from build123d import *
from build123d.topology import SkipClean

# Parameters (mm, degrees)
SKETCH_1_R          = 24.5
EXTRUDE_1_DEPTH     = 4.75
EXTRUDE_START       = 5.5
EXTRUDE_2_DEPTH     = 5.5
EXTRUDE_START_2     = 4.75
EXTRUDE_3_DEPTH     = 4.75
SKETCH_6_R          = 8.95
CUT_EXTRUDE_1_DEPTH = 38.755794257
SKETCH_8_W          = 30
SKETCH_8_H          = 10
EXTRUDE_4_DEPTH     = 5
FILLET_1_R          = 10
FILLET_2_R          = 5
MM_1_D              = 5
SKETCH_11_W         = 11.168523271
SKETCH_11_H         = 1.926491066
CUT_EXTRUDE_2_DEPTH = 45.650628903
CUT_EXTRUDE_3_DEPTH = 45.584890939
FILLET_3_R          = 2.5


# Some blends are built 0.0001 mm under size
with BuildPart() as part:
    # 草图1 → 凸台-拉伸1 (new body)
    with BuildSketch(Plane(origin=(0, 0, 0), x_dir=(1, 0, 0), z_dir=(0, 1, 0))):
        with Locations(Location((0, 0, 0), (0, 0, 270))):
            Circle(SKETCH_1_R)
    extrude(amount=EXTRUDE_1_DEPTH)

    # 草图4 → 凸台-拉伸2 (add)
    with BuildSketch(Plane.XZ.offset(EXTRUDE_START)):
        with BuildLine():
            Line((-23, 0), (-24.5, 0))
            ThreePointArc((-24.5, 0), (-22.635048547, 9.375744093), (-17.324116139, 17.324116139))
            Line((-17.324116139, 17.324116139), (-16.263455967, 16.263455967))
            ThreePointArc((-16.263455967, 16.263455967), (-21.249229248, 8.801718944), (-23, 0))
        make_face()
        with BuildLine():
            Line((23, 0), (24.5, 0))
            ThreePointArc((24.5, 0), (22.635048547, -9.375744093), (17.324116139, -17.324116139))
            Line((17.324116139, -17.324116139), (16.263455967, -16.263455967))
            ThreePointArc((16.263455967, -16.263455967), (21.249229248, -8.801718944), (23, 0))
        make_face()
    extrude(amount=-EXTRUDE_2_DEPTH)

    # 草图5 → 凸台-拉伸3 (add)
    with SkipClean():  # the faces are left unmerged after this step: merging them gives an invalid solid
        with BuildSketch(Plane.XZ.offset(5.5).offset(EXTRUDE_START_2)):
            with BuildLine():
                Line((-23, 0), (-24.5, 0))
                ThreePointArc((-24.5, 0), (-18.768088856, 15.748296437), (-4.254380353, 24.127789949))
                Line((-4.254380353, 24.127789949), (-3.993908086, 22.650578319))
                ThreePointArc((-3.993908086, 22.650578319), (-17.619022192, 14.784115023), (-23, 0))
            make_face()
            with BuildLine():
                Line((3.993908086, -22.650578319), (4.254380353, -24.127789949))
                ThreePointArc((4.254380353, -24.127789949), (18.768088856, -15.748296437), (24.5, 0))
                Line((24.5, 0), (23, 0))
                ThreePointArc((23, 0), (17.619022192, -14.784115023), (3.993908086, -22.650578319))
            make_face()
        extrude(amount=-EXTRUDE_3_DEPTH)

    # 草图6 → 切除-拉伸1 (cut, through all)
    with SkipClean():  # the faces are left unmerged after this step: merging them gives an invalid solid
        with BuildSketch(Plane(origin=(0, 4.75, 0), x_dir=(1, 0, 0), z_dir=(0, 1, 0))):
            with Locations(Location((0, 0, 0), (0, 0, 270))):
                Circle(SKETCH_6_R)
        extrude(amount=-CUT_EXTRUDE_1_DEPTH, mode=Mode.SUBTRACT)

    # 草图8 → 凸台-拉伸4 (add)
    with SkipClean():  # the faces are left unmerged after this step: merging them gives an invalid solid
        with BuildSketch(Plane(origin=(0, 0, 0), x_dir=(0.7071067811865489, 0, -0.7071067811865462), z_dir=(0.7071067811865462, 0, 0.7071067811865489))):
            with Locations((24.5, 9.75)):
                Rectangle(SKETCH_8_W, SKETCH_8_H)
        extrude(amount=EXTRUDE_4_DEPTH)

    # 圆角1
    fillet_1_edges = [part.edges().sort_by_distance(p)[0] for p in [
        (8.485281374, 14.75, -4.949747468),
    ]]
    fillet(fillet_1_edges, radius=FILLET_1_R - 0.0001)  # a hair under: the kernel refuses the full size

    # 圆角2
    fillet_2_edges = [part.edges().sort_by_distance(p)[0] for p in [
        (29.69848481, 14.75, -26.162950904),
        (29.69848481, 4.75, -26.162950904),
    ]]
    fillet(fillet_2_edges, radius=FILLET_2_R - 0.0001)  # a hair under: the kernel refuses the full size

    # 大小mm 暗销孔1 (through all)
    with Locations(Plane(origin=(3.535533906, 0, 3.535533906), x_dir=(0.7071067811865488, 0, -0.7071067811865462), z_dir=(0.7071067811865462, 0, 0.7071067811865488))):
        with Locations((32.49436991, 9.75)):
            Hole(MM_1_D / 2)

    # 草图11 → 切除-拉伸2 (cut, through all)
    with BuildSketch(Plane(origin=(3.535533906, 0, 3.535533906), x_dir=(0.7071067811865489, 0, -0.7071067811865461), z_dir=(0.7071067811865461, 0, 0.7071067811865489))):
        with Locations((29.568631546, 5.713245533)):
            Rectangle(SKETCH_11_W, SKETCH_11_H)
    extrude(amount=-CUT_EXTRUDE_2_DEPTH, mode=Mode.SUBTRACT)

    # 草图12 → 切除-拉伸3 (cut, through all)
    with BuildSketch(Plane(origin=(0, 0, 0), x_dir=(-0.7071067811865489, 0, 0.7071067811865461), z_dir=(-0.7071067811865461, 0, -0.7071067811865489))):
        with BuildLine():
            Line((-32.081510731, 14.75), (-9.5, 4.75))
            ThreePointArc((-9.5, 4.75), (-12.428932188, 11.821067812), (-19.5, 14.75))
            Line((-19.5, 14.75), (-32.081510731, 14.75))
        make_face()
    extrude(amount=-CUT_EXTRUDE_3_DEPTH, mode=Mode.SUBTRACT)


with BuildPart() as cut_extrude_3_kept_piece:
    # of the separate pieces the step leaves, the one the design keeps (cut_extrude_3_pieces_kept)
    add(part.part.solids().sort_by_distance((24.395254662, 14.75, -24.395254662))[0])

    # 圆角3
    # the kernel refuses this fillet: 2.5 mm, written as the material it takes off along each edge
    with BuildSketch(Plane(origin=(-16.75, -10.25, 0), x_dir=(0, 1, 0), z_dir=(-1, 0, 0)), Plane(origin=(2.908606976, -10.25, -16.495529863), x_dir=(0.9848077530122085, 0, 0.17364817766692725), z_dir=(0.17364817766692725, 0, -0.9848077530122086)), Plane(origin=(30.75, -10.25, 0), x_dir=(0, 0, -1), z_dir=(-1, 0, 0))) as fillet_3_piece_1:
        with BuildLine():
            CenterArc((FILLET_3_R, -FILLET_3_R), FILLET_3_R, 90, 90)
            Line((0, -FILLET_3_R), (0, 0))
            Line((0, 0), (FILLET_3_R, 0))
        make_face()
    extrude(amount=14, mode=Mode.SUBTRACT)
    with BuildSketch(Plane(origin=(2.908606976, -5.5, -16.495529863), x_dir=(0.9848077530122085, 0, 0.17364817766692725), z_dir=(0.17364817766692725, 0, -0.9848077530122086)), Plane(origin=(-5.339681463, -5.5, 30.282838405), x_dir=(0, -1, 0), z_dir=(0.17364817766692875, 0, -0.9848077530122084)), Plane(origin=(-5.339681463, -10.25, 30.282838405), x_dir=(-0.9848077530122084, 0, -0.17364817766692872), z_dir=(0.17364817766692875, 0, -0.9848077530122084))) as fillet_3_piece_2:
        with BuildLine():
            CenterArc((FILLET_3_R, FILLET_3_R), FILLET_3_R, 180, 90)
            Line((0, FILLET_3_R), (0, 0))
            Line((0, 0), (FILLET_3_R, 0))
        make_face()
    extrude(amount=14, mode=Mode.SUBTRACT)


solid = cut_extrude_3_kept_piece.part
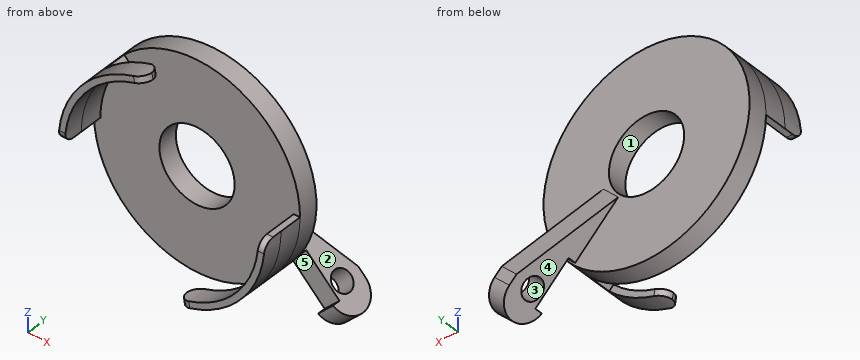
Part model, mm, in its own coordinate system. Face numbers are marked on the shaded views. A direction names the side the tool comes from. Give positions to 0.01 mm unless a question says otherwise; leave off trailing zeros. Loops run counter-clockwise (first coordinate to the right, second up) from the corner with the lowest first, then second, coordinate; pieces in that order, holes last. Notation, with made-up numbers: (22.5, -7) -> (41.5, -7) arc R36 ccw to (41.5, 27) -> close; hole circle Ø5 at (48.25, 1.25). An arc over 180 degrees is marked (long way). Write each question's results on one line, items separated by ' | '. Start each with the question number.
Q1. Band-saw the part on A-A on y = -2.25. List the corners of the cut face in (x, z), plus the area to 3 significant figures.
Q2. Band-saw the part on D-D on y = 1.5. List the corners of the cut face in (x, z).
Q3. Pull direction Z, two halves, no side cores. Call the marked faces 3, 4 and 5: +Z half, -Z half, draft (parallel to the pull), parting line (faces both ways), or undercut.
Q4. Wall check: L1, parallel to X at y = 3.8, z = 0; L2, parallel to Z at x = 0.5, y = 3.5; L3, parallel to Y at x = 18.5, z = -1. Give the ranges that are in metal, low to high.
Q5. Band-saw the part on C-C on x = 2. List the corners of the cut face in (y, z), plus the area to 3 significant figures.
Q6. Band-saw the part on B-B on z = 7. List the corners of the cut face in (x, y).
Q7. Which spindle directions (+Z, -Z, +X, -X, +Y, -Y) get a long thin tool onto all of the face, cutting with end or side? Do the marked faces 1 and 2. Say none if no direction does.
Q8. Pin check, flat tips, straight feed: P1, Ø24.5, axis at x = -0.5, z = 8.5, coming from the -Y side; P2, Ø2, axis at x = 14, z = -20.5, coming from the +Y side; P3, Ø12, axis at x = -13.5, y = -1, coming from the +Z side; P4, Ø10.5, axis at x = 0, z = 0, coming from the +Y side. Stop position of each tip, or through.
Results are:
1) outline: (-24.5, 0) -> (-23, 0) arc R23 cw to (-16.26, 16.26) -> (-17.32, 17.32) arc R24.5 ccw to start; (16.26, -16.26) -> (17.32, -17.32) arc R24.5 ccw to (24.5, 0) -> (23, 0) arc R23 cw to start | area: 56.0 mm²
2) outline: circle Ø49 at (0, 0); hole circle Ø17.9 at (0, 0)
3) face 3: undercut | face 4: -Z half | face 5: draft
4) L1: x = -24.5 to -8.95, 8.95 to 24.5 | L2: z = -24.49 to -8.94, 8.94 to 24.49 | L3: y = 0 to 4.75
5) outline: (0, -24.42) -> (4.75, -24.42) -> (4.75, -8.72) -> (0, -8.72) -> close; (0, 8.72) -> (4.75, 8.72) -> (4.75, 24.42) -> (0, 24.42) -> close | area: 149 mm²
6) outline: (-23.48, -10.25) -> (-21.91, -10.25) -> (-21.91, 0) -> (-5.58, 0) -> (-5.58, 4.75) -> (-23.48, 4.75) -> close; (5.58, 0) -> (23.48, 0) -> (23.48, 4.75) -> (5.58, 4.75) -> close
7) face 1: +Y, -Y | face 2: +Z, +X, +Y
8) P1: stops at y = 0 | P2: stops at y = 4.75 | P3: stops at z = 23.3 | P4: passes through
